Work out the finished part from the listing and answer in its coordinate system (mm). A direction names the side the tool comes from. Round coordinates to 2 decimals unless told otherwise and drop trailing zeros. Order: outer loops, then holes, each group sorted by start corner. A loop starts at its lowest first (then second) coordinate and runs counter-clockwise, first axis right, second up. Notation, with made-up numbers: M -16.5,52 L 30.5,52 A18 cw 30.5,66 Z; hole C 32,-39.75 d4. An arc over 180 degrees is marked long. Return JSON: item names as keys, results as strings.
from build123d import *

# Parameters (mm, degrees)
F1_DEPTH = 12.7
F3_D     = 6.35
F5_DEPTH = 12.701


with BuildPart() as f1:
    # F0 (on Top) → F1 (new body)
    with BuildSketch(Plane.XY):
        with BuildLine():
            Line((-57.44794, 20.666091), (-64.273439, 20.666091))
            Line((-64.273439, 20.666091), (-64.273439, -67.117393))
            Line((-64.273439, -67.117393), (-57.44794, -67.117393))
            Line((-57.44794, -67.117393), (-57.44794, -11.452466))
            ThreePointArc((-57.44794, -11.452466), (-50.363343, 5.745429), (-33.439308, 13.461399))
            Line((-33.439308, 13.461399), (1.706375, 13.461399))
            ThreePointArc((1.706375, 13.461399), (6.33048, 15.256632), (8.531871, 19.701751))
            Line((8.531871, 19.701751), (8.531871, 39.43621))
            ThreePointArc((8.531871, 39.43621), (5.119123, 42.332037), (1.706375, 39.43621))
            Line((1.706375, 39.43621), (1.706375, 20.666091))
            Line((1.706375, 20.666091), (-57.44794, 20.666091))
        make_face()
    extrude(amount=F1_DEPTH)

    # F3 (through all)
    with Locations(Plane(origin=(-64.273439, 0, 0), x_dir=(0, -1, 0), z_dir=(-1, 0, 0))):
        with Locations((-11.100469, 6.05725), (49.949814, 6.436449)):
            Hole(F3_D / 2)

    # F4 (on face) → F5 (cut, through all)
    with BuildSketch(Plane(origin=(0, 0, 0), x_dir=(1, 0, 0), z_dir=(0, 0, -1))):
        Polygon((-57.44794, 67.117393), (-64.273439, 67.117393), (-57.44794, 55.511292), align=None)
    extrude(amount=-F5_DEPTH, mode=Mode.SUBTRACT)


solid = f1.part
Item 1: The mould has two halves that part along Y. Classify faces 1 (the flat face through (-31, 20.666, 6)), 2 (the cylindrical face through (-44.56, 14.13, 7.01)), 3 (the cylindrical face through (-53.18, 2.25, 6.26)): pulls with the +Y half, pulls with the -Y half, needs draft (parallel to the pull), parting line crosses it, or undercut.
Output:
{"face 1": "pulls with the +Y half", "face 2": "undercut", "face 3": "pulls with the -Y half"}
Item 2: Find section B-B (z = 11). Determine the outline of the cut face in (x, y).
Output:
{"outline": "M -64.27,-67.12 L -57.45,-55.51 L -57.45,-11.45 A25.32 cw -33.44,13.46 L 1.71,13.46 A6.85 ccw 8.53,19.7 L 8.53,39.44 A3.46 ccw 1.71,39.44 L 1.71,20.67 L -64.27,20.67 Z"}
Item 3: Each of these flat-tipped pins is pushed along its axis until it touches: pin 1 (5 mm diameter, centred on x = -15.5, z = 3.5, fed in from -Y); pin 2 (6.5 mm diameter, centred on y = 33, z = 8.5, fed in from -X); pin 3 (6.5 mm diameter, centred on x = -27, z = 8.5, fed in from +Y). Where does it stop, or does it pass through?
Output:
{"pin 1": "stops at y = 13.46", "pin 2": "stops at x = 1.71", "pin 3": "stops at y = 20.67"}
Item 4: Which of the six approach directions +Z, -Z, +X, -X, +Y, -Y give full straight-line access (tool end or side, diameter ignored) to faces 4 (the cylindrical face through (5.19, 42.33, 6.26)), 5 (the flat face through (-16, 13.461, 2)), 6 (the flat face through (1.706, 30, 6))?
Output:
{"face 4": "+Z, -Z, +Y", "face 5": "+Z, -Z, +X, -Y", "face 6": "+Z, -Z, -X, +Y"}
Item 5: Find section A-A (x = -21). Determine the outline of the cut face in (y, z) (3 decimals).
Output:
{"outline": "M 13.461,0 L 20.666,0 L 20.666,12.7 L 13.461,12.7 L 13.461,8.18 A3.175 cw 13.461,3.934 Z"}
Item 6: Find section D-D (z = 5). Determine the outline of the cut face in (x, y), plus the area to 3 significant figures.
Output:
{"outline": "M -64.27,-67.12 L -57.45,-55.51 L -57.45,-52.78 L -64.27,-52.78 Z; M -64.27,-47.12 L -57.45,-47.12 L -57.45,-11.45 A25.32 cw -47.75,8.11 L -64.27,8.11 Z; M -64.27,14.09 L 4.58,14.09 A6.85 ccw 8.53,19.7 L 8.53,39.44 A3.46 ccw 1.71,39.44 L 1.71,20.67 L -64.27,20.67 Z", "area": "1,110 mm^2"}
Item 7: Consider line 1 along Y through (x, z) = (-58, 4.5); line 2 along Y through (x, z) = (-31, 2); line 3 along X through (y, z) = (-21.5, 10.75). Determine where each line is inside the solid, lowest interval first. Write a range as [from, to].
Output:
{"line 1": "y = [-56.45, -52.47], [-47.43, 8.33], [13.87, 20.67]", "line 2": "y = [13.46, 20.67]", "line 3": "x = [-64.27, -57.45]"}
Item 8: Find section C-C (x = -51). Determine the outline of the cut face in (y, z) (3 decimals).
Output:
{"outline": "M 5.06,0 L 20.666,0 L 20.666,12.7 L 5.06,12.7 Z; hole C 11.1,6.057 d6.35"}
